Geometry check sheet. Reference: drawing and pictorial views, mm from the part's lowest x, y, z. A direction names the side the tool comes from. Coordinates: 2 decimals unless noted, no trailing zeros. Loops run counter-clockwise (first coordinate to the right, second up) from the corner with the lowest first, then second, coordinate; pieces in that order, holes last.
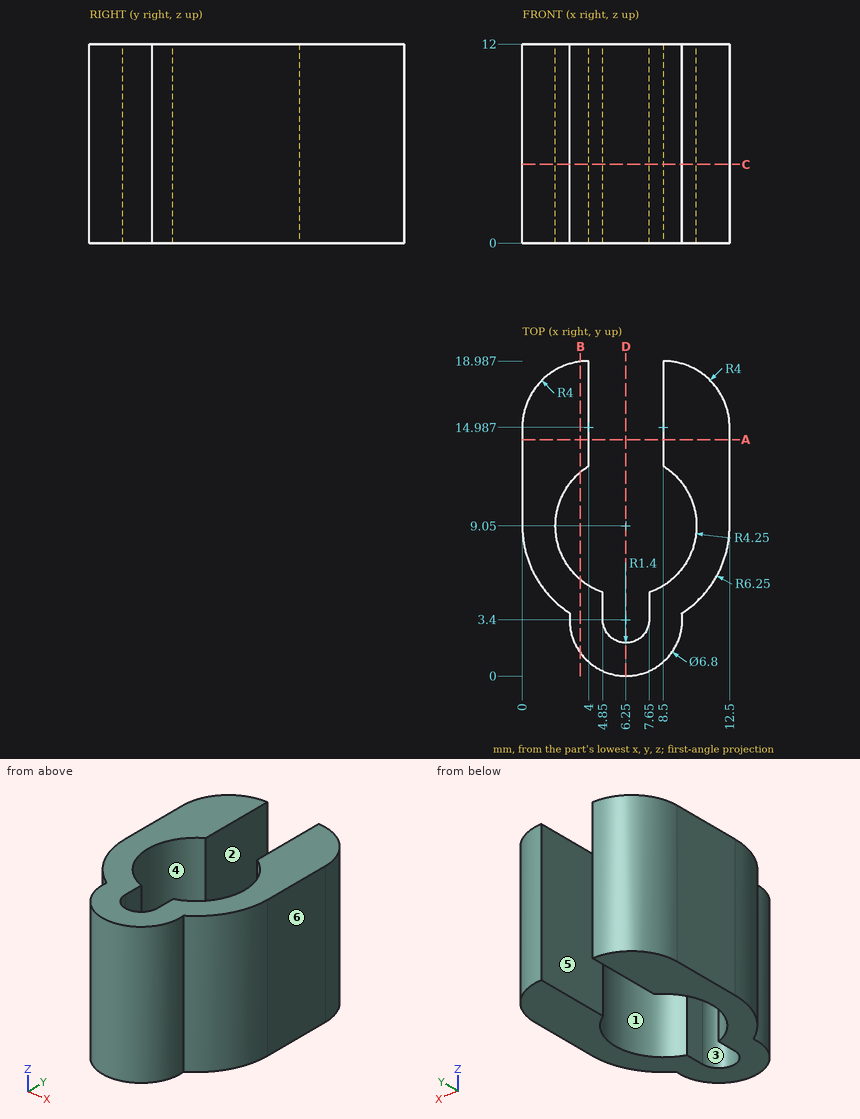
1) Section check A-A on y = 14.25. Record the cut outline in (x, z), and give its area (3 significant figures).
Data:
outline: (0, 0) - (4, 0) - (4, 12) - (0, 12) - close; (8.5, 0) - (12.5, 0) - (12.5, 12) - (8.5, 12) - close
area: 96.0 mm2
2) Mould release check, pull along Y, two halves, no side actions. Record for the marked faces 1, 2 and 3: +Y half, -Y half, draft (parallel to the pull), parting line (faces both ways), or undercut.
Data:
face 1: undercut
face 2: draft
face 3: +Y half
3) Material ranges on probe 1 along X at (y, z) = (8.5, 6); probe 2 along X at (y, z) = (7.75, 5.75); probe 3 along Y at (x, z) = (2.75, 5.5) (1 decimal), recorded low to high.
Data:
probe 1: x = 0.02 to 2.04, 10.46 to 12.48
probe 2: x = 0.14 to 2.2, 10.3 to 12.36
probe 3: y = 3.9 to 6.6, 11.5 to 18.8
4) Depth check by flat-ended pin: pin 1 (0.8 mm diameter, centred on y = 4, z = 7.5, fed in from +X); pin 2 (0.5 mm diameter, centred on y = 4.5, z = 5.5, fed in from -X) (1 decimal); pin 3 (1 mm diameter, centred on y = 8.5, z = 9.5, fed in from +X); pin 4 (4 mm diameter, centred on y = 3, z = 7, fed in from +X). Enter the tip coordinate at first touch or a pass-through.
Data:
pin 1: stops at x = 10.43
pin 2: stops at x = 1.7
pin 3: stops at x = 12.5
pin 4: stops at x = 11.01
5) Section check B-B on x = 3.5. Record the cut outline in (y, z), and give its area (3 significant figures).
Data:
outline: (1.4, 0) - (5.81, 0) - (5.81, 12) - (1.4, 12) - close; (12.29, 0) - (18.96, 0) - (18.96, 12) - (12.29, 12) - close
area: 133 mm2
6) Access from +Z, -Z, +X, -X, +Y, -Y to the whole of each face (thin tool, end or side, straight path). Record for the marked faces 4, 5 and 6.
Data:
face 4: +Z, -Z
face 5: +Z, -Z, +Y
face 6: +Z, -Z, +X, +Y, -Y
7) Section check D-D on x = 6.25. Record the cut outline in (y, z).
Data:
outline: (0, 0) - (2, 0) - (2, 12) - (0, 12) - close
8) Section check C-C on z = 4.75. Record the cut outline in (x, y).
Data:
outline: (0, 9.05) arc R6.25 ccw to (2.87, 3.79) arc R3.4 ccw (long way) to (9.63, 3.79) arc R6.25 ccw to (12.5, 9.05) - (12.5, 14.99) arc R4 ccw to (8.5, 18.99) - (8.5, 12.66) arc R4.25 cw to (7.65, 5.04) - (7.65, 3.4) arc R1.4 cw to (4.85, 3.4) - (4.85, 5.04) arc R4.25 cw to (4, 12.66) - (4, 18.99) arc R4 ccw to (0, 14.99) - close
